Design review of the part built by this model. Coordinates are the model's own, in mm. A direction names the side the tool comes from. Coordinates: 2 decimals unless noted, no trailing zeros. Loops run counter-clockwise (first coordinate to the right, second up) from the corner with the lowest first, then second, coordinate; pieces in that order, holes last. Notation, with made-up numbers: (45, 8) - (91, 8) arc R18 ccw to (91, 38) - close; hole circle Ø7 at (34.5, -17.5). An arc over 180 degrees is marked (long way). Use one line per item in the form item = value. Start each with the question number.
(1) Add section C-C (x = 3). State the section outline as (y, z) points, plus the area to 3 significant figures.
(2) Add section D-D (z = 50). State the section outline as (x, y) points.
(3) Add section B-B (y = -12). State the section outline as (x, z) points, plus the area to 3 significant figures.
(4) For L1, parallel to Z at x = 10, y = 0; L2, parallel to Y at x = 13.25, z = 37.5; L3, parallel to Z at x = 1.25, y = 17.5, list the stretches that pass through material, from the lowest coordinate up.
(5) Tool access review of faces 4 (the face through (7, 7, 14)), 5 (the face through (7, -7, 15)), 6 (the face through (9.93, 0.651, 42.457)): name each direction out of +Z, -Z, +X, -X, +Y, -Y from which nothing blocks a thin tool from reaching the whole face with its end or side.
(6) The part is to be moulded in two halves that separate along Y. For faces 1 (the face through (7, 17, 4)), 2 (the face through (15, -1, 28)), 3 (the face through (2.52, -0.19, 36.65)), say which applies: pulls with the +Y half, pulls with the -Y half, needs draft (parallel to the pull), parting line crosses it, or undercut.
(7) Add section A-A (x = 7.25). State the section outline as (y, z) points.
(8) Clearance check with flat-ended pins moving along their axes: pin 1 Ø2 at (x, z) = (12, 6.5) entering from +Y; pin 2 Ø6 at (y, z) = (7, 44.5) entering from -X; pin 3 Ø7 at (x, z) = (4, 6) entering from -Y. State where each tip first meets the part, or that it passes through.
```python
from build123d import *

# Parameters (mm, degrees)
F1_DEPTH = 15
F3_D     = 10
F3_DEPTH = 10
F3_TIP   = 3.0043030951


with BuildPart() as f1:
    # F0 (on Right) → F1 (new body)
    with BuildSketch(Plane.YZ):
        Polygon((-7, 9), (-17, 9), (-17, 0), (17, 0), (17, 9), (7, 9), (7, 20), (-7, 20), align=None)
        with BuildLine():
            Line((-45, 20), (-7, 20))
            Line((-7, 20), (7, 20))
            Line((7, 20), (45, 20))
            Line((45, 20), (45, 40))
            Line((45, 40), (32.3431457505, 52.6568542495))
            ThreePointArc((32.3431457505, 52.6568542495), (29.7477589599, 54.3910362601), (26.686291501, 55))
            Line((26.686291501, 55), (-26.686291501, 55))
            ThreePointArc((-26.686291501, 55), (-29.7477589599, 54.3910362601), (-32.3431457505, 52.6568542495))
            Line((-32.3431457505, 52.6568542495), (-45, 40))
            Line((-45, 40), (-45, 20))
        make_face()
    extrude(amount=F1_DEPTH)

    # F3
    with Locations(Plane.YZ.offset(15)):
        with Locations((0, 37.5)):
            Hole(F3_D / 2, depth=F3_DEPTH)
            with Locations((0, 0, -(F3_DEPTH + F3_TIP / 2))):  # 118° drill point
                Cone(0, F3_D / 2, F3_TIP, mode=Mode.SUBTRACT)


solid = f1.part
```
Computed values:
q1.outline = (-45, 20) - (-7, 20) - (-7, 9) - (-17, 9) - (-17, 0) - (17, 0) - (17, 9) - (7, 9) - (7, 20) - (45, 20) - (45, 40) - (32.34, 52.66) arc R8 ccw to (26.69, 55) - (-26.69, 55) arc R8 ccw to (-32.34, 52.66) - (-45, 40) - close; hole circle Ø3.34 at (0, 37.5)
q1.area = 3,370 mm^2
q2.outline = (0, -35) - (15, -35) - (15, 35) - (0, 35) - close
q3.outline = (0, 0) - (15, 0) - (15, 9) - (0, 9) - close; (0, 20) - (15, 20) - (15, 55) - (0, 55) - close
q3.area = 660 mm^2
q4.L1 = 0 to 32.5, 42.5 to 55
q4.L2 = -45 to -5, 5 to 45
q4.L3 = 20 to 55
q5.face_4 = +X, -X, +Y
q5.face_5 = +X, -X, -Y
q5.face_6 = +X
q6.face_1 = pulls with the +Y half
q6.face_2 = needs draft
q6.face_3 = undercut
q7.outline = (-45, 20) - (-7, 20) - (-7, 9) - (-17, 9) - (-17, 0) - (17, 0) - (17, 9) - (7, 9) - (7, 20) - (45, 20) - (45, 40) - (32.34, 52.66) arc R8 ccw to (26.69, 55) - (-26.69, 55) arc R8 ccw to (-32.34, 52.66) - (-45, 40) - close; hole circle Ø10 at (0, 37.5)
q8.pin_1 = 17
q8.pin_2 = 0
q8.pin_3 = -17
